CAD build for the part. Positions are in the model's coordinates, mm. A direction names the side the tool comes from. Round coordinates to 2 decimals unless told otherwise and drop trailing zeros. Order: outer loops, then holes, each group sorted by start corner. A loop starts at its lowest first (then second) coordinate and runs counter-clockwise, first axis right, second up. Notation, with made-up numbers: (-18.75, 3.5) -> (-4.75, 3.5) arc R13 cw to (-4.75, 25.5) -> close; hole circle Ø2 at (7.5, -28.75). An arc over 180 degrees is marked (long way). Return JSON: item names as keys, results as strings. Group by question number.
Q1. Which spindle directions (+Z, -Z, +X, -X, +Y, -Y) get a long thin tool onto all of the face, cutting with end or side? Do faces 1 (the cylindrical face through (6.373, -84.29, -10.527)), 2 (the flat face through (10, 6, -27.5)), 3 (the flat face through (10, 5, -17.5)), 4 (the flat face through (5, -87, -10)), 5 (the cylindrical face through (17.54, 1.43, -9)). Say none if no direction does.
Q2. Cut at B-B (x = 8.5). Write the cut outline in (y, z).
Q3. Probe line 1 along Y through (x, z) = (2.8, -12.5); line 2 along Y through (x, z) = (2, -12.5); line 3 along Z through (x, y) = (3.9, 5). List the from-to ranges inside material, lowest first.
Q4. Flat gauge pins, fed straight in: pin 1 (2.5 mm diameter, centred on x = 6.5, y = -86.5, fed in from +Z); pin 2 (3 mm diameter, centred on y = 3.5, z = -13.5, fed in from -X); pin 3 (5 mm diameter, centred on x = 12, y = -40, fed in from +Z); pin 4 (1.8 mm diameter, centred on y = -88, z = 1.5, fed in from -X). Where does each tip first touch, or does it go through?
Q5. Mould opens along Y. For faces 6 (the flat face through (5, 5, -16)), 7 (the cylindrical face through (17.54, 8.5, -8.93)), 8 (the cylindrical face through (2.54, 1.43, -9)) say: +Y half, -Y half, draft (parallel to the pull), parting line (faces both ways), or undercut.
Q6. Cut at C-C (x = 13.5). Write the cut outline in (y, z).
from build123d import *

# Parameters (mm, degrees)
SKETCH3_W               = 20
SKETCH3_H               = 10
BOSS_EXTRUDE2_DEPTH     = 20
CUT_EXTRUDE2_REACH      = 37.444
SKETCH4_W               = 10
SKETCH4_H               = 10
CUT_EXTRUDE3_DEPTH      = 33.882366095
CUT_EXTRUDE3_DEPTH_BACK = 33.882366095
SKETCH5_R               = 2.5
BOSS_EXTRUDE3_DEPTH     = 20
BOSS_EXTRUDE4_START     = -10
BOSS_EXTRUDE4_DEPTH     = 10
CUT_EXTRUDE4_DEPTH      = 10
FILLET1_R               = 5
FILLET2_R               = 2.5


with BuildPart() as part:
    # Sketch3 → Boss-Extrude2 (new body)
    with BuildSketch(Plane(origin=(0, 0, 0), x_dir=(0, 0, -1), z_dir=(1, 0, 0))):
        with Locations((17.5, 5)):
            Rectangle(SKETCH3_W, SKETCH3_H)
    extrude(amount=BOSS_EXTRUDE2_DEPTH)

    # Sketch4 → Cut-Extrude2 (cut, up to next)
    with BuildSketch(Plane(origin=(0, 10, 0), x_dir=(1, 0, 0), z_dir=(0, 1, 0)), mode=Mode.PRIVATE) as cut_extrude2_sk1:
        with Locations((10, 12.5)):
            Rectangle(SKETCH4_W, SKETCH4_H)
    cut_extrude2_tool1 = extrude(cut_extrude2_sk1.sketch, amount=-CUT_EXTRUDE2_REACH, mode=Mode.PRIVATE) & part.part
    add(cut_extrude2_tool1.solids().sort_by_distance((10, 10, -12.5))[0], mode=Mode.SUBTRACT)

    # Sketch5 → Cut-Extrude3 (cut, two sides: drawn at the far end of the back side and taken through both)
    with BuildSketch(Plane(origin=(5, 0, 0), x_dir=(0, 0, -1), z_dir=(1, 0, 0)).offset(-CUT_EXTRUDE3_DEPTH_BACK)):
        with Locations((12.5, 5)):
            Circle(SKETCH5_R)
    extrude(amount=CUT_EXTRUDE3_DEPTH + CUT_EXTRUDE3_DEPTH_BACK, mode=Mode.SUBTRACT)

    # Sketch6 → Boss-Extrude3 (add)
    with BuildSketch(Plane(origin=(0, 0, 0), x_dir=(0, 0, -1), z_dir=(1, 0, 0))):
        with BuildLine():
            Line((0, -85), (0, -90))
            ThreePointArc((0, -90), (47.895258826, -54.354239164), (27.5, 1.758232721))
            Line((27.5, 1.758232721), (20.615528128, 0))
            ThreePointArc((20.615528128, 0), (43.732139211, -50.606601718), (0, -85))
        make_face()
    extrude(amount=BOSS_EXTRUDE3_DEPTH)

    # Sketch7 → Boss-Extrude4 (add)
    with BuildSketch(Plane(origin=(20, 0, 0), x_dir=(0, 0, -1), z_dir=(1, 0, 0)).offset(BOSS_EXTRUDE4_START)):
        with BuildLine():
            Line((0, -85), (0, -90))
            ThreePointArc((0, -90), (-5.0254481, -89.74680765), (-10, -88.989794856))
            Line((-10, -88.989794856), (-10, -83.874821937))
            ThreePointArc((-10, -83.874821937), (-5.031551095, -84.717820761), (0, -85))
        make_face()
    extrude(amount=BOSS_EXTRUDE4_DEPTH)

    # Sketch8 → Cut-Extrude4 (cut)
    with BuildSketch(Plane.ZY):
        with BuildLine():
            Line((0, -85), (0, -90))
            ThreePointArc((0, -90), (-5.0254481, -89.74680765), (-10, -88.989794856))
            Line((-10, -88.989794856), (-10, -83.874821937))
            ThreePointArc((-10, -83.874821937), (-5.031551095, -84.717820761), (0, -85))
        make_face()
    extrude(amount=-CUT_EXTRUDE4_DEPTH, mode=Mode.SUBTRACT)

    # Fillet1
    fillet1_edges = [part.edges().sort_by_distance(p)[0] for p in [
        (17.5, 0, -7.5),
        (17.5, 10, -7.5),
        (2.5, 10, -7.5),
        (2.5, 0, -7.5),
    ]]
    fillet(fillet1_edges, radius=FILLET1_R - 0.0001)  # a hair under: the kernel refuses the full size

    # Fillet2
    fillet2_edges = [part.edges().sort_by_distance(p)[0] for p in [
        (20, -55.429880165, -42.271962317),
        (0, -45.650302702, -44.643858249),
        (10, -85, 0),
        (15, -83.874821937, 10),
        (5, -83.874821937, -10),
    ]]
    fillet(fillet2_edges, radius=FILLET2_R)


solid = part.part
Solution:
{
 "1": {"face 1": "+Z, -X", "face 2": "-Z, +X, -X, +Y", "face 3": "+Z, +Y", "face 4": "+Z, -X, -Y", "face 5": "+Z, +X, -X"},
 "2": {"outline": "(-88.99, -10) arc R50 ccw to (1.76, -27.5) -> (10, -27.5) -> (10, -17.5) -> (0, -17.5) -> (0, -20.62) arc R45 cw to (-83.41, -11.84) arc R2.5 ccw to (-85.83, -10) -> close"},
 "3": {"line 1": "y = -88.41 to -83.23, 0 to 2.5, 7.5 to 10", "line 2": "y = -88.41 to -83.28, 0 to 2.5, 7.5 to 10", "line 3": "z = -27.5 to -15, -10 to -7.5"},
 "4": {"pin 1": "stops at z = -10", "pin 2": "stops at x = 0", "pin 3": "stops at z = -44.93", "pin 4": "stops at x = 10"},
 "5": {"face 6": "draft", "face 7": "+Y half", "face 8": "undercut"},
 "6": {"outline": "(-88.99, 10) arc R50 ccw to (1.76, -27.5) -> (10, -27.5) -> (10, -17.5) -> (0, -17.5) -> (0, -20.62) arc R45 cw to (-84.44, 7.11) arc R2.5 ccw to (-86.9, 10) -> close"}
}
